Input: part model. Units: mm. Frame: model coordinates. Round coordinates to 2 decimals unless told otherwise and drop trailing zeros. Order: outer loops, then holes, each group sorted by start corner. A loop starts at its lowest first (then second) coordinate and runs counter-clockwise, first axis right, second up. Notation, with made-up numbers: (18.5, 44.5) - (72.5, 44.5) arc R26 cw to (72.5, 61.5) - close; hole circle Ø1 at (34.5, 13.5). An arc over 180 degrees is marked (long way). One line per item, written item: value. Start each with the question number.
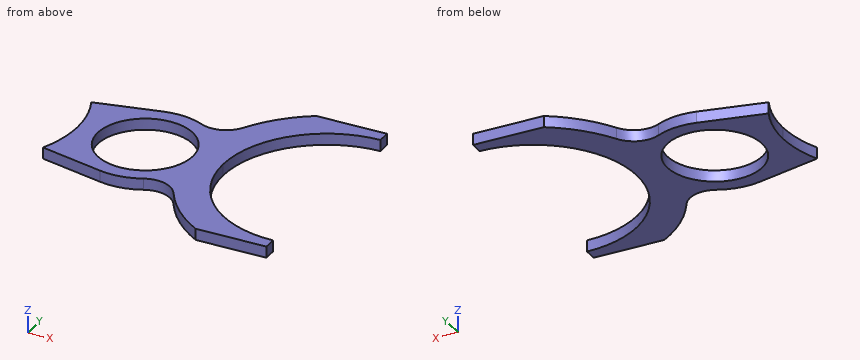
from build123d import *

# Parameters (mm, degrees)
MODEL_R             = 8.375
BOSS_EXTRUDE1_DEPTH = 2


with BuildPart() as part:
    # Model → Boss-Extrude1 (new body)
    with BuildSketch(Plane.XY):
        with BuildLine():
            Line((74.448010934, 2.249927661), (74.448004895, 4.500084718))
            Line((74.448004895, 4.500084718), (61.968150916, 4.500005388))
            ThreePointArc((61.968150916, 4.500005388), (57.22880439, 0.718152869), (53.588491837, -4.130758193))
            ThreePointArc((53.588491837, -4.130758193), (50.805713706, -6.36868051), (47.244750466, -6.10092834))
            ThreePointArc((47.244750466, -6.10092834), (43.728043409, -5.074712325), (40.069365021, -5.260239392))
            Line((40.069365021, -5.260239392), (28.682107763, -7.782293479))
            ThreePointArc((28.682107763, -7.782293479), (30.001771143, -11.797316195), (30.448277219, -16.000000001))
            ThreePointArc((30.448277219, -16.000000001), (30.001771143, -20.202683806), (28.682107763, -24.217706522))
            Line((28.682107763, -24.217706522), (40.069365021, -26.73976061))
            ThreePointArc((40.069365021, -26.73976061), (43.728043409, -26.925287677), (47.244750466, -25.899071661))
            ThreePointArc((47.244750466, -25.899071661), (50.805713706, -25.631319491), (53.588491837, -27.869241808))
            ThreePointArc((53.588491837, -27.869241808), (57.22880439, -32.718152871), (61.968150916, -36.500005389))
            Line((61.968150916, -36.500005389), (74.448004895, -36.500084719))
            Line((74.448004895, -36.500084719), (74.448010934, -34.249927662))
            ThreePointArc((74.448010934, -34.249927662), (61.543360309, -28.904678271), (56.198007214, -16.000070602))
            ThreePointArc((56.198007214, -16.000070602), (61.543310386, -3.095371653), (74.448010934, 2.249927661))
        make_face()
        with Locations((42.448007213, -15.999981536)):
            Circle(MODEL_R, mode=Mode.SUBTRACT)
    extrude(amount=BOSS_EXTRUDE1_DEPTH)


solid = part.part
Item 1: Section query A-A on y = -22. Return loops of the section in (x, z).
Item 2: First-contact query: pin 1 Ø6 at (x, y) = (57.5, -17.5) entering from +Z. Flat tip, straight axial feed; report the tip coordinate or a pass-through.
Item 3: Section query B-B on x = 66. Return loops of the section in (y, z).
Item 4: Section query D-D on x = 54.5. Return loops of the section in (y, z).
Item 5: Line query: L1, parallel to Y at x = 48.5, z = 1.25; L2, parallel to Y at x = 69.5, z = 1.7; L3, parallel to X at y = -9, z = 0.6. Output: solid intervals per line, ascending.
Geometry results:
1. outline: (29.53, 0) - (36.61, 0) - (36.61, 2) - (29.53, 2) - close; (48.29, 0) - (57.21, 0) - (57.21, 2) - (48.29, 2) - close
2. pin 1: stops at z = 2
3. outline: (-36.5, 0) - (-32.18, 0) - (-32.18, 2) - (-36.5, 2) - close; (0.18, 0) - (4.5, 0) - (4.5, 2) - (0.18, 2) - close
4. outline: (-29.34, 0) - (-2.66, 0) - (-2.66, 2) - (-29.34, 2) - close
5. L1: y = -25.49 to -21.79, -10.21 to -6.51
5. L2: y = -36.5 to -33.57, 1.57 to 4.5
5. L3: x = 29.18 to 37.85, 47.05 to 57.59
